from build123d import *

# Parameters (mm, degrees)
F0_W     = 37.110798
F0_H     = 33.024196
F1_DEPTH = 200
F2_R     = 18.630211
F3_DEPTH = 100


with BuildPart() as f1:
    # F0 (on Top) → F1 (new body)
    with BuildSketch(Plane.XY):
        with Locations((18.555399, 16.512098)):
            Rectangle(F0_W, F0_H)
        Polygon((29.538543, 14.172093), (23.027837, 6.007926), (12.585476, 6.007926), (6.07477, 14.172093), (8.398414, 24.352643), (17.806657, 28.883413), (27.214899, 24.352643), align=None, mode=Mode.SUBTRACT)
    extrude(amount=F1_DEPTH)

    # F2 (on face) → F3 (join)
    with BuildSketch(Plane(origin=(0, 33.024196, 0), x_dir=(-1, 0, 0), z_dir=(0, 1, 0))):
        with Locations((-21.135863, 32.111328)):
            Circle(F2_R)
    extrude(amount=-F3_DEPTH)


solid = f1.part
Design review of the part built by this model. Coordinates are the model's own, in mm. A direction names the side the tool comes from. Coordinates: 2 decimals unless noted, no trailing zeros. Write each loop counter-clockwise with the first axis right and the second up, starting at its lowest first coordinate (ties: lowest second). Pieces come first, ordered by that corner, then holes. Notation, with made-up numbers: (60.25, 54.5) - (108.25, 54.5) arc R10 ccw to (108.25, 63.5) - close; hole circle Ø9 at (44, -15.5). An arc over 180 degrees is marked (long way). One line per item, written item: value.
1) Add section D-D (y = 19). State the section outline as (x, z) points, plus the area to 3 significant figures.
Answer sheet:
outline: (0, 0) - (7.18, 0) - (7.18, 19.77) arc R18.63 ccw to (28.44, 14.97) - (28.44, 0) - (37.11, 0) - (37.11, 22.53) arc R18.63 ccw to (37.11, 41.7) - (37.11, 200) - (28.44, 200) - (28.44, 49.25) arc R18.63 ccw to (7.18, 44.45) - (7.18, 200) - (0, 200) - close
area: 3,940 mm2
2) Add section C-C (x = 25). State the section outline as (y, z) points.
Answer sheet:
outline: (-66.98, 13.89) - (0, 13.89) - (0, 0) - (8.48, 0) - (8.48, 13.89) - (25.42, 13.89) - (25.42, 0) - (33.02, 0) - (33.02, 200) - (25.42, 200) - (25.42, 50.34) - (8.48, 50.34) - (8.48, 200) - (0, 200) - (0, 50.34) - (-66.98, 50.34) - close
3) For faces 1 (the face through (22.44, 26.65, 7.15)), 2 (the face through (37.111, 16, 120)), 3 (the face through (13.04, 26.59, 121.77)), list the 3-axis set-ups (+Z, -Z, +X, -X, +Y, -Y) from which the entire face can be reached by the end or side of a thin tool; tool diameter is ignored.
Answer sheet:
face 1: -Z
face 2: +Z, +X, +Y, -Y
face 3: +Z
4) Add section B-B (y = 8.5). State the section outline as (x, z) points.
Answer sheet:
outline: (0, 0) - (10.6, 0) - (10.6, 16.75) arc R18.63 ccw to (25.02, 13.89) - (25.02, 0) - (37.11, 0) - (37.11, 22.53) arc R18.63 ccw to (37.11, 41.7) - (37.11, 200) - (25.02, 200) - (25.02, 50.33) arc R18.63 ccw to (10.6, 47.47) - (10.6, 200) - (0, 200) - close
5) To check wall thickness, follow probe 1 along Y at (x, z) = (16, 176); probe 2 along X at (y, z) = (7, 65); probe 3 along Z at (x, y) = (21, 24). State the ranges of each line that lie inside material, in increasing order.
Answer sheet:
probe 1: y = 0 to 6.01, 28.01 to 33.02
probe 2: x = 0 to 11.79, 23.82 to 37.11
probe 3: z = 13.48 to 50.74
6) Add section A-A (z = 106). State the section outline as (x, y) points, plus the area to 3 significant figures.
Answer sheet:
outline: (0, 0) - (37.11, 0) - (37.11, 33.02) - (0, 33.02) - close; hole (6.07, 14.17) - (12.59, 6.01) - (23.03, 6.01) - (29.54, 14.17) - (27.21, 24.35) - (17.81, 28.88) - (8.4, 24.35) - close
area: 829 mm2
7) Insertion check: pin 1 (18.5 mm diameter, centred on x = 18, z = 99, fed in from -Y); pin 2 (8 mm diameter, centred on x = 34.5, y = -23.5, fed in from -Z); pin 3 (8 mm diameter, centred on x = 24.5, y = 6, fed in from -Z); pin 4 (1 mm diameter, centred on x = 26, y = -31.5, fed in from -Z). Each pin has a flat end and moves straight along its axis. Give the tip position at first contact, or say it passes through.
Answer sheet:
pin 1: stops at y = 0
pin 2: stops at z = 16.01
pin 3: stops at z = 0
pin 4: stops at z = 14
